The listing builds one solid part. Answer for the finished solid, in the listing's coordinates (mm). Give positions to 0.01 mm unless a question says otherwise; leave off trailing zeros. Loops run counter-clockwise (first coordinate to the right, second up) from the corner with the lowest first, then second, coordinate; pieces in that order, holes last. Notation, with made-up numbers: M 42,74 L 87,74 A33 cw 87,106 Z; hole C -33,-2.5 d11. An arc over 180 degrees is marked long. Use one line per item in the form item = value. Start each with the question number.
1. The part is cut by section B-B (z = 11.5). Write down the section's boundary in (x, y) (3 decimals).
2. Straight lines are drawn through the part: line 1 (X direction, y = 2.2, z = 0) (3 decimals); line 2 (Z direction, x = 0, y = 1.95); line 3 (X direction, y = 2.25, z = 7) (3 decimals). For each, find the intervals that lie inside material, in ascending order. Write a range as from..to.
3. The part is cut by section D-D (x = 24.5). Write down the section's boundary in (y, z) (3 decimals).
4. The part is cut by section C-C (x = 0). Write down the section's boundary in (y, z) (3 decimals).
5. Each of these flat-tipped pins is pushed along its axis until it touches: pin 1 Ø1.1 at (y, z) = (1.5, -42) entering from -X; pin 2 Ø1 at (x, y) = (-23, 0.5) entering from -Z (3 decimals); pin 3 Ø0.6 at (x, y) = (30.5, 2) entering from +Z (3 decimals). Where does it stop, or does it pass through?
6. The part is cut by section A-A (z = 0). Write down the section's boundary in (x, y) (3 decimals).
from build123d import *

# Parameters (mm, degrees)
BOSS_EXTRUDE1_DEPTH = 3.175
SKETCH2_R           = 6.5
SKETCH2_W           = 3.175
SKETCH2_H           = 30
CUT_EXTRUDE1_DEPTH  = 4.175
FILLET1_R           = 1


with BuildPart() as part:
    # Sketch1 → Boss-Extrude1 (new body)
    with BuildSketch(Plane(origin=(0, 0, 0), x_dir=(1, 0, 0), z_dir=(0, 1, 0))):
        Polygon((-38.1, -40.925), (-10, -40.925), (-10, -44.1), (10, -44.1), (10, -40.925), (38.1, -40.925), (38.1, 40.925), (10, 40.925), (10, 44.1), (-10, 44.1), (-10, 40.925), (-38.1, 40.925), align=None)
    extrude(amount=BOSS_EXTRUDE1_DEPTH)

    # Sketch2 → Cut-Extrude1 (cut, through all)
    with BuildSketch(Plane(origin=(0, 3.175, 0), x_dir=(1, 0, 0), z_dir=(0, 1, 0))):
        Circle(SKETCH2_R)
        with Locations((30.1625, 0)):
            Rectangle(SKETCH2_W, SKETCH2_H)
    extrude(amount=-CUT_EXTRUDE1_DEPTH, mode=Mode.SUBTRACT)

    # Fillet1
    fillet1_edges = [part.edges().sort_by_distance(p)[0] for p in [
        (10, 1.5875, 44.1),
        (-10, 1.5875, 44.1),
        (-10, 1.5875, -44.1),
        (10, 1.5875, -44.1),
        (28.575, 1.5875, 15),
        (28.575, 1.5875, -15),
        (31.75, 1.5875, -15),
        (31.75, 1.5875, 15),
    ]]
    fillet(fillet1_edges, radius=FILLET1_R)


solid = part.part
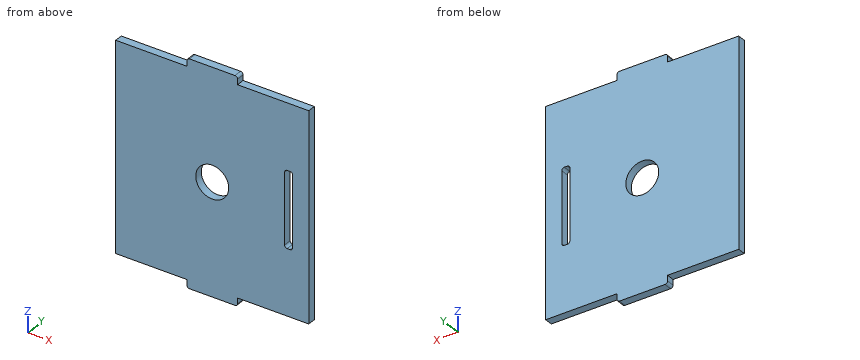
Derived:
q1.outline = M -38.1,0 L 28.575,0 L 28.575,3.175 L -38.1,3.175 Z; M 31.75,0 L 38.1,0 L 38.1,3.175 L 31.75,3.175 Z
q2.line_1 = -38.1..-6.5, 6.5..28.575, 31.75..38.1
q2.line_2 = -44.1..-6.5, 6.5..44.1
q2.line_3 = -38.1..28.575, 31.75..38.1
q3.outline = M 0,-40.925 L 3.175,-40.925 L 3.175,40.925 L 0,40.925 Z
q4.outline = M 0,-44.1 L 3.175,-44.1 L 3.175,-6.5 L 0,-6.5 Z; M 0,6.5 L 3.175,6.5 L 3.175,44.1 L 0,44.1 Z
q5.pin_1 = -10
q5.pin_2 = -40.925
q5.pin_3 = 40.925
q6.outline = M -38.1,0 L -6.5,0 L -6.5,3.175 L -38.1,3.175 Z; M 6.5,0 L 28.575,0 L 28.575,3.175 L 6.5,3.175 Z; M 31.75,0 L 38.1,0 L 38.1,3.175 L 31.75,3.175 Z
